```python
from build123d import *

# Parameters (mm, degrees)
F1_W     = 53
F1_H     = 55
F1_W_2   = 43
F1_H_2   = 45
F2_DEPTH = 35
F1_R     = 6.116576
F3_DEPTH = 10


with BuildPart() as f2:
    # F1 (on face) → F2 (new body)
    with BuildSketch(Plane.XZ):
        with Locations((-19.479784, 2.733284)):
            Rectangle(F1_W, F1_H)
        with Locations((-19.305006, 2.440175)):
            Rectangle(F1_W_2, F1_H_2, mode=Mode.SUBTRACT)
    extrude(amount=F2_DEPTH)

    # F1 (on face) → F3 (join)
    with BuildSketch(Plane.XZ):
        with Locations((-19.305006, 2.440175)):
            Rectangle(F1_W_2, F1_H_2)
        with Locations((-18.968696, 4.535152)):
            Circle(F1_R, mode=Mode.SUBTRACT)
    extrude(amount=F3_DEPTH)


solid = f2.part
```
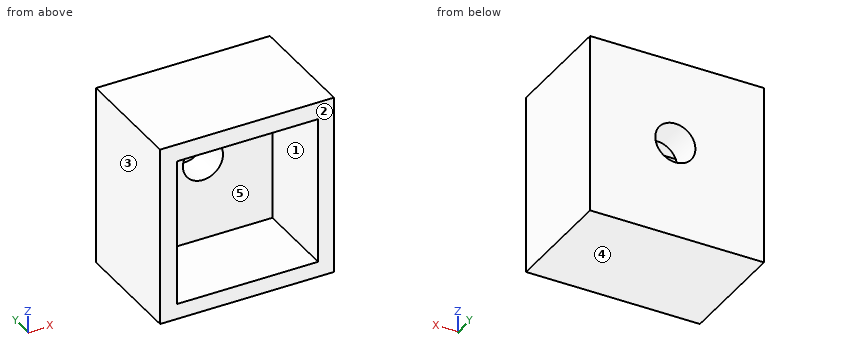
Check sheet for the modelled part. Datum: model origin and axes. Units: mm. Face numbers are marked on the shaded views. A direction names the side the tool comes from. Coordinates: 2 decimals unless noted, no trailing zeros. Write each loop counter-clockwise with the first axis right and the second up, starting at its lowest first coordinate (ties: lowest second). Pieces come first, ordered by that corner, then holes. Notation, with made-up numbers: (58, -29) -> (68, -29) arc R34 cw to (68, 2) -> close; hole circle Ø1 at (31, 18). An arc over 180 degrees is marked (long way). Use a Markdown table: item, result.
1. Sectioned sample at B-B (x = -31.5). Enter the section's corners in (y, z), plus the area to 3 significant figures.
Reported:
| item | result |
|---|---|
| outline | (-35, -24.77) -> (0, -24.77) -> (0, 30.23) -> (-35, 30.23) -> (-35, 24.94) -> (-10, 24.94) -> (-10, -20.06) -> (-35, -20.06) -> close |
| area | 800 mm2 |
2. Release check for a two-part mould opening along Z. For the marked faces 3, 4 and 5 record: pulls with the +Z half, pulls with the -Z half, needs draft (parallel to the pull), parting line crosses it, or undercut.
Reported:
| item | result |
|---|---|
| face 3 | needs draft |
| face 4 | pulls with the -Z half |
| face 5 | undercut |
3. Tool access check on the marked faces 1 and 2. Record the directions out of +Z, -Z, +X, -X, +Y, -Y that give a thin tool (end or side, any length) a straight path to the whole face; none if there is none.
Reported:
| item | result |
|---|---|
| face 1 | -Y |
| face 2 | +Z, -Z, +X, -X, -Y |
4. Go/stop test with a flat-tipped pin: pin 1 Ø11 at (x, z) = (-18.97, 4.54) entering from +Y. Record where the tip stops, or that it passes through.
Reported:
| item | result |
|---|---|
| pin 1 | passes through |
5. Sectioned sample at D-D (z = 18). Enter the section's corners in (x, y) (3 decimals).
Reported:
| item | result |
|---|---|
| outline | (-45.98, -35) -> (-40.805, -35) -> (-40.805, -10) -> (2.195, -10) -> (2.195, -35) -> (7.02, -35) -> (7.02, 0) -> (-45.98, 0) -> close |
6. Sectioned sample at C-C (z = 6.5). Enter the section's corners in (x, y) (3 decimals), plus the area to 3 significant figures.
Reported:
| item | result |
|---|---|
| outline | (-45.98, -35) -> (-40.805, -35) -> (-40.805, -10) -> (-24.761, -10) -> (-24.761, 0) -> (-45.98, 0) -> close; (-13.176, -10) -> (2.195, -10) -> (2.195, -35) -> (7.02, -35) -> (7.02, 0) -> (-13.176, 0) -> close |
| area | 664 mm2 |
7. Sectioned sample at A-A (y = -16.5). Enter the section's corners in (x, z) (3 decimals), plus the area to 3 significant figures.
Reported:
| item | result |
|---|---|
| outline | (-45.98, -24.767) -> (7.02, -24.767) -> (7.02, 30.233) -> (-45.98, 30.233) -> close; hole (-40.805, -20.06) -> (2.195, -20.06) -> (2.195, 24.94) -> (-40.805, 24.94) -> close |
| area | 980 mm2 |
8. Scan lines: line 1 along Z through (x, y) = (-24, -11); line 2 along X through (y, z) = (-18, 17.5) (3 decimals); line 3 along Y through (x, z) = (-36.5, 13). Record each from-to range of solid material in increasing order.
Reported:
| item | result |
|---|---|
| line 1 | z = -24.77 to -20.06, 24.94 to 30.23 |
| line 2 | x = -45.98 to -40.805, 2.195 to 7.02 |
| line 3 | y = -10 to 0 |
